Input: part model. Units: mm. Frame: model coordinates. A direction names the side the tool comes from. Give positions to 0.01 mm unless a question says otherwise; leave off trailing zeros. Order: outer loops, then holes, each group sorted by start corner. A loop starts at its lowest first (then second) coordinate and runs counter-clockwise, first axis right, second up. Notation, with made-up numbers: (24, 26) - (44, 26) arc R27 ccw to (44, 57) - close; hole circle Ø5 at (9.5, 84.5). An arc over 180 degrees is marked (long way). Answer in a Markdown table with one row per item. Add a question column.
1. Section query A-A on y = 0. Return loops of the section in (x, z), and give its area (3 significant figures).
2. Contact query for flat-ended pins moving along their axis: pin 1 (10 mm diameter, centred on x = 49.5, z = 5, fed in from +Y); pin 2 (1.5 mm diameter, centred on y = 57, z = 15, fed in from -X); pin 3 (8 mm diameter, centred on y = 13.5, z = 6.5, fed in from -X). Output: stop coordinate, or through.
3. Ray query, line 1 (Y direction, x = 1.5, z = 14.5); line 2 (Y direction, x = 0, z = 0.3); line 3 (Z direction, x = -58, y = -45). Return the intervals inside material, ascending. Write a range as [from, to].
4. Access query for faces 1 (the face through (-58.85, -45.12, 0.38)), 2 (the face through (-69.01, 3.04, 25.02)), 3 (the face through (-11.671, -52.557, 12.672)). Directions: +Z, -Z, +X, -X, +Y, -Y. A direction counts if a zero-diameter tool reaches every point of the face in a straight line with its end or side. Return the directions, or none.
5. Mould query, pull axis X, two halves, no side actions, for faces 4 (the face through (25.184, -48.419, 10.153)), 5 (the face through (-19.38, -87.27, 12.67)), 6 (the face through (-69.01, 3.04, 0.38)). Classes: released by +X, released by -X, zero draft, split by the parting line, or undercut.
```python
from build123d import *

# Parameters (mm, degrees)
F0_R       = 89.3972749213
F0_R_2     = 53.8372732699
F1_DEPTH   = 25.4
F2_SIZE2   = 10.6711628823
F2_SIZE    = 15.24
F2_2_SIZE2 = 10.6711628823
F2_2_SIZE  = 15.24
F3_DEPTH   = 0.762
F4_DEPTH   = 0.762


with BuildPart() as f1:
    # F0 (on Top) → F1 (new body)
    with BuildSketch(Plane.XY):
        Circle(F0_R)
        Circle(F0_R_2, mode=Mode.SUBTRACT)
    extrude(amount=F1_DEPTH)

    # F2
    f2_edges = [f1.edges().sort_by_distance(p)[0] for p in [
        (-89.397275, 0, 25.4),
        (-53.837273, 0, 25.4),
    ]]
    f2_side = f1.faces().sort_by_distance((-86.868738, 0, 25.4))[0]
    chamfer(f2_edges, length=F2_SIZE, length2=F2_SIZE2, reference=f2_side)

    # F2#2
    f2_2_edges = [f1.edges().sort_by_distance(p)[0] for p in [
        (-89.397275, 0, 0),
        (-53.837273, 0, 0),
    ]]
    f2_2_side = f1.faces().sort_by_distance((-86.868738, 0, 0))[0]
    chamfer(f2_2_edges, length=F2_2_SIZE, length2=F2_2_SIZE2, reference=f2_2_side)

    # F3 (cut): faces of the model
    f3_faces = [f1.faces().sort_by_distance(p)[0] for p in [
        (-72.0597904424, 0, 25.4),
        (-72.0597904424, 0, 0),
    ]]
    extrude(f3_faces, amount=-F3_DEPTH, dir=(0, 0, 1), mode=Mode.SUBTRACT)

    # F4 (cut): a face of the model
    f4_faces = [f1.faces().sort_by_distance(p)[0] for p in [
        (-72.0597904424, 0, 0),
    ]]
    extrude(f4_faces, amount=-F4_DEPTH, mode=Mode.SUBTRACT)


solid = f1.part
```
Answer:
| question | item | result |
|---|---|---|
| 1 | outline | (-89.4, 10.67) - (-74.16, 0) - (-74.16, 0.76) - (-69.08, 0.76) - (-69.08, 0) - (-53.84, 10.67) - (-53.84, 14.73) - (-69.08, 25.4) - (-69.08, 24.64) - (-74.16, 24.64) - (-74.16, 25.4) - (-89.4, 14.73) - close; (53.84, 10.67) - (69.08, 0) - (69.08, 0.76) - (74.16, 0.76) - (74.16, 0) - (89.4, 10.67) - (89.4, 14.73) - (74.16, 25.4) - (74.16, 24.64) - (69.08, 24.64) - (69.08, 25.4) - (53.84, 14.73) - close |
| 1 | area | 1,140 mm² |
| 2 | pin 1 | stops at y = 73.9 |
| 2 | pin 2 | stops at x = -69.44 |
| 2 | pin 3 | stops at x = -88.16 |
| 3 | line 1 | y = [-89.38, -53.82], [53.82, 89.38] |
| 3 | line 2 | y = [-74.59, -74.16], [-69.08, -68.65], [68.65, 69.08], [74.16, 74.59] |
| 3 | line 3 | z = [0.76, 24.64] |
| 4 | face 1 | -Z |
| 4 | face 2 | +Z |
| 4 | face 3 | +Z, -Z |
| 5 | face 4 | undercut |
| 5 | face 5 | split by the parting line |
| 5 | face 6 | undercut |
